from build123d import *

# Parameters (mm, degrees)
CUERPO_PROFILE_R                     = 15
BRIDA_IZQ_PROFILE_R                  = 25
BRIDA_DCHA_PROFILE_R                 = 25
TALADRO_EJE_PROFILE_R                = 5
ALOJAMIENTO_RODAMIENTO_IZQ_PROFILE_R = 13


with BuildPart() as part:
    # Cuerpo: sweep along a curve in space
    with BuildLine() as cuerpo_path:
        Line((-425.1, 65, -50), (-425.1, 65, 25.5))
    # Cuerpo profile (on start of the path) → Cuerpo (sweep)
    with BuildSketch(Plane(origin=(-425.1, 65, -50), x_dir=(1, 0, 0), z_dir=(0, 0, 1))):
        Circle(CUERPO_PROFILE_R)
    sweep(path=cuerpo_path.line)

    # Brida_izq: sweep along a curve in space
    with BuildLine() as brida_izq_path:
        Line((-425.1, 65, -44.5), (-425.1, 65, -41.5))
    # Brida_izq profile (on start of the path) → Brida_izq (sweep)
    with BuildSketch(Plane(origin=(-425.1, 65, -44.5), x_dir=(1, 0, 0), z_dir=(0, 0, 1))):
        Circle(BRIDA_IZQ_PROFILE_R)
    sweep(path=brida_izq_path.line)

    # Brida_dcha: sweep along a curve in space
    with BuildLine() as brida_dcha_path:
        Line((-425.1, 65, 22.5), (-425.1, 65, 25.5))
    # Brida_dcha profile (on start of the path) → Brida_dcha (sweep)
    with BuildSketch(Plane(origin=(-425.1, 65, 22.5), x_dir=(1, 0, 0), z_dir=(0, 0, 1))):
        Circle(BRIDA_DCHA_PROFILE_R)
    sweep(path=brida_dcha_path.line)

    # Taladro_eje: sweep along a curve in space
    with BuildLine() as taladro_eje_path:
        Line((-425.1, 65, -50), (-425.1, 65, 25.5))
    # Taladro_eje profile (on start of the path) → Taladro_eje (sweep, cut)
    with BuildSketch(Plane(origin=(-425.1, 65, -50), x_dir=(1, 0, 0), z_dir=(0, 0, 1))):
        Circle(TALADRO_EJE_PROFILE_R)
    sweep(path=taladro_eje_path.line, mode=Mode.SUBTRACT)

    # Alojamiento_rodamiento_izq: sweep along a curve in space
    with BuildLine() as alojamiento_rodamiento_izq_path:
        Line((-425.1, 65, -50), (-425.1, 65, -42))
    # Alojamiento_rodamiento_izq profile (on start of the path) → Alojamiento_rodamiento_izq (sweep, cut)
    with BuildSketch(Plane(origin=(-425.1, 65, -50), x_dir=(1, 0, 0), z_dir=(0, 0, 1))):
        Circle(ALOJAMIENTO_RODAMIENTO_IZQ_PROFILE_R)
    sweep(path=alojamiento_rodamiento_izq_path.line, mode=Mode.SUBTRACT)


solid = part.part
Here's how the part is built. I have some questions about the finished solid (model axes, mm). A direction names the side the tool comes from. Give positions to 0.01 mm unless a question says otherwise; leave off trailing zeros. Write each loop counter-clockwise with the first axis right and the second up, starting at its lowest first coordinate (ties: lowest second). Pieces come first, ordered by that corner, then holes. Notation, with made-up numbers: (-1.75, -20) -> (26.25, -20) arc R12 cw to (26.25, -8) -> close; hole circle Ø1 at (-28, -28). An arc over 180 degrees is marked (long way). Use one line per item in the form item = value. Start each with the question number.
1. Imagine slicing it at C-C on z = 0.5. List the corners of the cut face in (x, y) for me, plus the area to 3 significant figures.
2. Imagine slicing it at B-B on x = -425.1. List the corners of the cut face in (y, z) for me.
3. Imagine slicing it at D-D on y = 85. List the corners of the cut face in (x, z) for me.
4. On a 3-axis mill with a long thin cutter (end or side, diameter ignored), from which of +Z, -Z, +X, -X, +Y, -Y can I reach the whole of each face in a straight line? I mean faces 1 (the face through (-425.2, 78.4, -50)), 2 (the face through (-414, 54, -41.5)), 3 (the face through (-412.7, 68.9, -45.9)). Say none if no direction works.
5. Will these pins go through, and if not, where does the flat tip stop? pin 1 Ø3 at (x, z) = (-431.5, -9.5) entering from +Y; pin 2 Ø1 at (y, z) = (69.5, -16) entering from -X; pin 3 Ø1 at (y, z) = (68.5, -35.5) entering from +X; pin 4 Ø9 at (x, y) = (-425.1, 65) entering from -Z.
6. Imagine slicing it at A-A on y = 65. List the corners of the cut face in (x, z) for me.
7. If I drill on L1, parallel to Z at x = -439, y = 55.5; L2, parallel to Y at x = -425.1, z = -47; L3, parallel to Y at x = -425, z = 4, over which ranges is the centre line in solid material (lowest first)?
8. Thinking about a two-plate mould opening in Y: for faces 4 (the face through (-444.94, 49.79, -42.98)), 5 (the face through (-420.33, 66.5, -7.78)), 6 (the face through (-425.4, 59.8, 25.5)), which applies, +Y half, -Y half, draft (parallel to the pull), parting line (faces both ways), or undercut?
Entries:
q1.outline = circle Ø30 at (-425.1, 65); hole circle Ø10 at (-425.1, 65)
q1.area = 628 mm²
q2.outline = (40, -44.5) -> (50, -44.5) -> (50, -50) -> (52, -50) -> (52, -42) -> (60, -42) -> (60, 25.5) -> (40, 25.5) -> (40, 22.5) -> (50, 22.5) -> (50, -41.5) -> (40, -41.5) -> close; (70, -42) -> (78, -42) -> (78, -50) -> (80, -50) -> (80, -44.5) -> (90, -44.5) -> (90, -41.5) -> (80, -41.5) -> (80, 22.5) -> (90, 22.5) -> (90, 25.5) -> (70, 25.5) -> close
q3.outline = (-440.1, -44.5) -> (-410.1, -44.5) -> (-410.1, -41.5) -> (-440.1, -41.5) -> close; (-440.1, 22.5) -> (-410.1, 22.5) -> (-410.1, 25.5) -> (-440.1, 25.5) -> close
q4.face_1 = -Z, +X, -X, +Y, -Y
q4.face_2 = none
q4.face_3 = -Z
q5.pin_1 = 79.18
q5.pin_2 = -439.56
q5.pin_3 = -410.4
q5.pin_4 = through
q6.outline = (-450.1, -44.5) -> (-440.1, -44.5) -> (-440.1, -50) -> (-438.1, -50) -> (-438.1, -42) -> (-430.1, -42) -> (-430.1, 25.5) -> (-450.1, 25.5) -> (-450.1, 22.5) -> (-440.1, 22.5) -> (-440.1, -41.5) -> (-450.1, -41.5) -> close; (-420.1, -42) -> (-412.1, -42) -> (-412.1, -50) -> (-410.1, -50) -> (-410.1, -44.5) -> (-400.1, -44.5) -> (-400.1, -41.5) -> (-410.1, -41.5) -> (-410.1, 22.5) -> (-400.1, 22.5) -> (-400.1, 25.5) -> (-420.1, 25.5) -> close
q7.L1 = -44.5 to -41.5, 22.5 to 25.5
q7.L2 = 50 to 52, 78 to 80
q7.L3 = 50 to 60, 70 to 80
q8.face_4 = parting line
q8.face_5 = undercut
q8.face_6 = draft
